Build history of the part. All positions in model axes, mm. Round coordinates to 2 decimals unless told otherwise and drop trailing zeros. Loops run counter-clockwise (first coordinate to the right, second up) from the corner with the lowest first, then second, coordinate; pieces in that order, holes last. Notation, with made-up numbers: (45.25, -34) - (59.25, -34) arc R23 ccw to (59.25, 4) - close; hole circle Ø6 at (53, 62). An arc over 180 degrees is marked (long way). Use one line per item in the form item = value. Start each with the question number.
Q1. Pin check, flat tips, straight feed: pin 1 (3 mm diameter, centred on x = 4.5, y = -4, fed in from +Z); pin 2 (1.5 mm diameter, centred on x = 6.5, z = 164.5, fed in from -Y); pin 3 (3 mm diameter, centred on x = 6.5, y = -5.5, fed in from -Z). Stop position of each tip, or through.
Q2. Drill centre lines: line 1 (Z direction, x = 8, y = 1.75); line 2 (Z direction, x = 4.5, y = -4.75); line 3 (Y direction, x = 9.25, z = 291.5). Where is each one in solid material? Low to high.
Q3. Saw through at A-A (y = -3.75). Give the cut face in (x, z) (3 decimals), then the cut area to 3 significant figures.
Q4. Saw through at C-C (x = 7.5). Give the cut face in (y, z), then the cut area to 3 significant figures.
Autodesk Inventor part; units mm, degrees
ref_plane "YZ Plane" through (0, 0, 0) normal (1, 0, 0) x (0, 1, 0)
ref_plane "XZ Plane" through (0, 0, 0) normal (0, 1, 0) x (-1, 0, 0)
ref_plane "XY Plane" through (0, 0, 0) normal (0, 0, 1) x (1, 0, 0)
sketch "Sketch1" plane through (0, 0, 0) normal (1, 0, 0) x (0, 1, 0)
  line L0 (-9.1281, -449.2848) -> (9.1281, -449.2848) construction
  line L1 (9.1281, -449.2848) -> (9.1281, 449.2848)
  line L2 (9.1281, 449.2848) -> (-9.1281, 449.2848) construction
  line L3 (-9.1281, 449.2848) -> (-9.1281, -449.2848)
  line L4 (-9.1281, -449.2848) -> (9.1281, 449.2848) construction
  line L5 (9.1281, -449.2848) -> (-9.1281, 449.2848) construction
  line L6 (-9.1281, 449.2848) -> (9.1281, 433.966)
  line L7 (-9.1281, -449.2848) -> (9.1281, -433.966)
  point P0 (0, 0)
  dimension "d0" = 898.5697
  dimension "d1" = 18.2563
  dimension "d16" = 40
  dimension "d17" = 40
extrude "Extrusion1" add sketch "Sketch1" along normal blind 9.525
chamfer "Chamfer1" distance 9.525 angle 11.388 1 edges at (9.525, -9.1281, 0) measured on face at (3.175, -9.1281, 149.7616)
sketch "Sketch4" plane through (0, -9.1281, -449.2848) normal (0.1975, -0.9803, 0) x (0.9803, 0.1975, 0)
  line L0 (0, 880.8231) -> (12.9422, 880.8231)
  line L1 (12.9422, 880.8231) -> (12.9422, 863.3606)
  line L2 (12.9422, 863.3606) -> (0, 863.3606)
  line L3 (0, 863.3606) -> (0, 880.8231)
  line L4 (12.9422, 15.3188) -> (12.9422, 883.2508)
  line L5 (0, 898.5697) -> (0, 0)
  point P0 (1.8024, 449.2848)
  dimension "d21" = 17.7466
  dimension "d22" = 17.4625
extrude "Extrusion4" cut sketch "Sketch4" against normal blind 9.525
mirror "Mirror2" about plane through (0, 0, 0) normal (0, 0, 1) of "Extrusion4"
properties part number "BASE_SIDEK_TREBUCHET" material "Wood (Birch)"
Report:
q1.pin_1 = 446.24
q1.pin_2 = -7.97
q1.pin_3 = -447.5
q2.line_1 = -440.16 to -431.54, -414.08 to 414.08, 431.54 to 440.16
q2.line_2 = -445.61 to -431.54, -414.08 to 414.08, 431.54 to 445.61
q2.line_3 = -7.27 to 9.13
q3.outline = (0, -444.772) - (9.525, -444.772) - (9.525, -431.538) - (0, -431.538) - close; (0, -414.076) - (9.525, -414.076) - (9.525, 414.076) - (0, 414.076) - close; (0, 431.538) - (9.525, 431.538) - (9.525, 444.772) - (0, 444.772) - close
q3.area = 8,140 mm²
q4.outline = (-7.62, -448.02) - (9.13, -433.97) - (9.13, 433.97) - (-7.62, 448.02) - (-7.62, 431.54) - (2.1, 431.54) - (2.1, 414.08) - (-7.62, 414.08) - (-7.62, -414.08) - (2.1, -414.08) - (2.1, -431.54) - (-7.62, -431.54) - close
q4.area = 14,400 mm²
